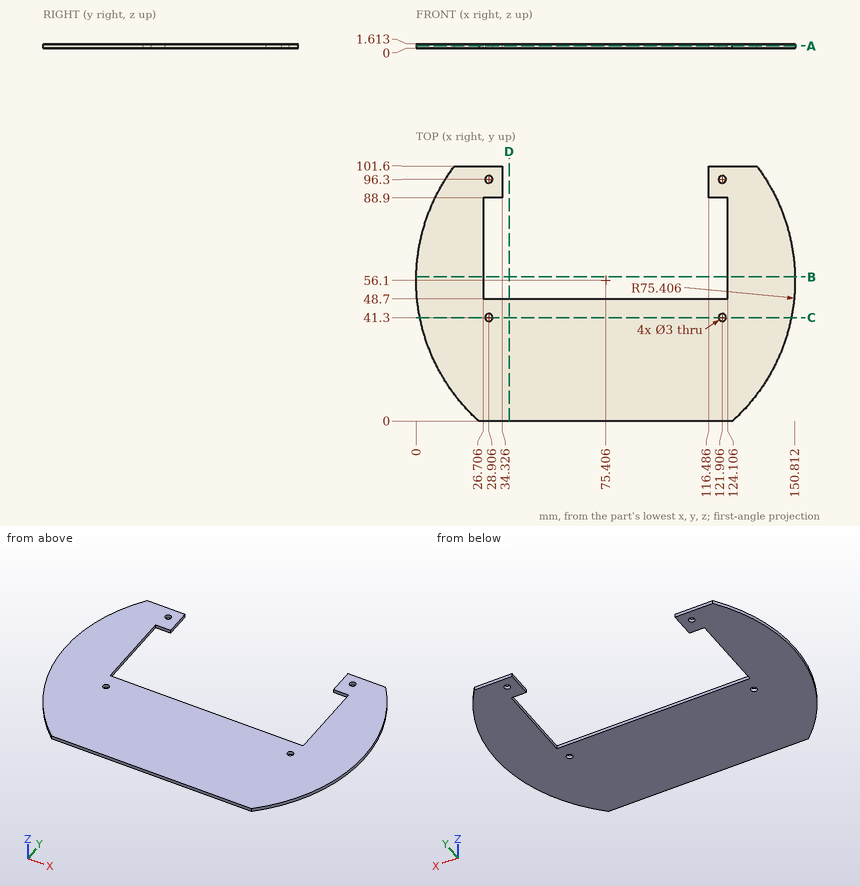
Geometry check sheet. Reference: drawing and pictorial views, mm from the part's lowest x, y, z. Round coordinates to 2 decimals unless told otherwise and drop trailing zeros. Loops run counter-clockwise (first coordinate to the right, second up) from the corner with the lowest first, then second, coordinate; pieces in that order, holes last. Notation, with made-up numbers: (87, 27) -> (135, 27) arc R27 ccw to (135, 48) -> close; hole circle Ø11 at (23.5, 62.5). An arc over 180 degrees is marked (long way). Answer as a JSON object with one key per item and string values.
Q1. Section check B-B (y = 57.5). Record the boundary of the cut face in (x, z).
Data:
{"outline": "(0.01, 0) -> (26.71, 0) -> (26.71, 1.61) -> (0.01, 1.61) -> close; (124.11, 0) -> (150.8, 0) -> (150.8, 1.61) -> (124.11, 1.61) -> close"}
Q2. Section check A-A (z = 0.9). Record the boundary of the cut face in (x, y) (1 decimal), then the cut area to 3 significant figures.
Data:
{"outline": "(15.3, 101.6) arc R75.4 ccw to (25, 0) -> (125.8, 0) arc R75.4 ccw to (135.5, 101.6) -> (116.5, 101.6) -> (116.5, 88.9) -> (124.1, 88.9) -> (124.1, 48.7) -> (26.7, 48.7) -> (26.7, 88.9) -> (34.3, 88.9) -> (34.3, 101.6) -> close; hole circle Ø3 at (28.9, 41.3); hole circle Ø3 at (28.9, 96.3); hole circle Ø3 at (121.9, 41.3); hole circle Ø3 at (121.9, 96.3)", "area": "9,030 mm2"}
Q3. Go/stop test with flat-tipped pins: P1, Ø1.8, axis at x = 28.91, y = 41.3, coming from the -Z side; P2, Ø0.8, axis at y = 75.5, z = 0.5, coming from the -X side; P3, Ø0.8, axis at x = 95, z = 0.5, coming from the +Y side; P4, Ø0.5, axis at y = 71.5, z = 1, coming from the +X side (1 decimal). Record where each tip stops, or that it passes through.
Data:
{"P1": "passes through", "P2": "stops at x = 2.43", "P3": "stops at y = 48.7", "P4": "stops at x = 149.3"}
Q4. Scan lines: line 1 (X direction, y = 96.3, z = 0.75) (1 decimal); line 2 (Y direction, x = 43, z = 1.15); line 3 (X direction, y = 68, z = 0.3) (1 decimal). Record each from-to range of solid material in increasing order. Write a range as from..to.
Data:
{"line 1": "x = 11.6..27.4, 30.4..34.3, 116.5..120.4, 123.4..139.2", "line 2": "y = 0..48.7", "line 3": "x = 0.9..26.7, 124.1..149.9"}
Q5. Section check D-D (x = 37). Record the boundary of the cut face in (y, z).
Data:
{"outline": "(0, 0) -> (48.7, 0) -> (48.7, 1.61) -> (0, 1.61) -> close"}
Q6. Section check C-C (y = 41.3). Record the boundary of the cut face in (x, z) (1 decimal), then the cut area to 3 significant figures.
Data:
{"outline": "(1.5, 0) -> (27.4, 0) -> (27.4, 1.6) -> (1.5, 1.6) -> close; (30.4, 0) -> (120.4, 0) -> (120.4, 1.6) -> (30.4, 1.6) -> close; (123.4, 0) -> (149.3, 0) -> (149.3, 1.6) -> (123.4, 1.6) -> close", "area": "229 mm2"}
